Read the model definition and answer for the solid it produces. Units are mm, in the model's axes. A direction names the side the tool comes from. Give positions to 0.01 mm unless a question says otherwise; leave off trailing zeros. Order: outer loops, then holes, each group sorted by start corner. A loop starts at its lowest first (then second) coordinate and runs counter-clockwise, first axis right, second up. Notation, with made-up numbers: M 66,-30.5 L 110,-30.5 A12 ccw 110,-12.5 Z; hole C 62.25,-39 d1. An arc over 180 degrees is marked long. One line per item, written item: value.
from build123d import *

# Parameters (mm, degrees)
SKETCH2_W                                    = 325
SKETCH2_H                                    = 220
SKETCH2_R                                    = 5
BOSS_EXTRUDE3_DEPTH                          = 15
SKETCH11_W                                   = 70
SKETCH11_H                                   = 90
SKETCH11_W_2                                 = 50
SKETCH11_H_2                                 = 75
CUT_EXTRUDE6_DEPTH                           = 5
FILLET1_R                                    = 5
CSK_FOR_M4_COUNTERSUNK_FLAT_HEAD_SCR_2_COUNT = 2
CSK_FOR_M4_COUNTERSUNK_FLAT_HEAD_SCR_2_PITCH = 100
CSK_FOR_M4_COUNTERSUNK_FLAT_HEAD_SCR_3_COUNT = 2
CSK_FOR_M4_COUNTERSUNK_FLAT_HEAD_SCR_3_PITCH = 202.484567313
CSK_FOR_M4_COUNTERSUNK_FLAT_HEAD_SCR_4_COUNT = 2
CSK_FOR_M4_COUNTERSUNK_FLAT_HEAD_SCR_4_PITCH = 236.008474424
CSK_FOR_M4_COUNTERSUNK_FLAT_HEAD_SCR_5_COUNT = 2
CSK_FOR_M4_COUNTERSUNK_FLAT_HEAD_SCR_5_PITCH = 232.594066992
CSK_FOR_M4_COUNTERSUNK_FLAT_HEAD_SCR_6_COUNT = 2
CSK_FOR_M4_COUNTERSUNK_FLAT_HEAD_SCR_6_PITCH = 210
M5_TAPPED_HOLE2_D                            = 4.2
M5_TAPPED_HOLE2_DEPTH                        = 5
M5_TAPPED_HOLE2_TIP                          = 1.2618073
M6_TAPPED_HOLE3_D                            = 5
M6_TAPPED_HOLE3_DEPTH                        = 5
M6_TAPPED_HOLE3_TIP                          = 1.502151548


with BuildPart() as part:
    # Sketch2 → Boss-Extrude3 (new body)
    with BuildSketch(Plane(origin=(0, 0, 0), x_dir=(1, 0, 0), z_dir=(0, 1, 0))):
        with Locations((7.596919738, 0)):
            Rectangle(SKETCH2_W, SKETCH2_H)
        with Locations(Location((155.096919738, -95, 0), (0, 0, 270))):
            Circle(SKETCH2_R, mode=Mode.SUBTRACT)
        with Locations(Location((155.096919738, 95, 0), (0, 0, 270))):
            Circle(SKETCH2_R, mode=Mode.SUBTRACT)
        with Locations(Location((-104.903080262, -95, 0), (0, 0, 270))):
            Circle(SKETCH2_R, mode=Mode.SUBTRACT)
        with Locations(Location((-104.903080262, 95, 0), (0, 0, 90))):
            Circle(SKETCH2_R, mode=Mode.SUBTRACT)
    extrude(amount=-BOSS_EXTRUDE3_DEPTH)

    # Sketch11 → Cut-Extrude6 (cut)
    with BuildSketch(Plane.XZ.offset(15)):
        with Locations((40.096919738, -50)):
            Rectangle(SKETCH11_W, SKETCH11_H)
        with Locations((-39.903080262, -50)):
            Rectangle(SKETCH11_W, SKETCH11_H)
        with Locations((-109.903080262, -42.5)):
            Rectangle(SKETCH11_W_2, SKETCH11_H_2)
        with Locations((-109.903080262, 42.5)):
            Rectangle(SKETCH11_W_2, SKETCH11_H_2)
        with Locations((-39.903080262, 50)):
            Rectangle(SKETCH11_W, SKETCH11_H)
        with Locations((40.096919738, 50)):
            Rectangle(SKETCH11_W, SKETCH11_H)
        Polygon((85.096919738, 95), (135.096919738, 95), (140.096919738, 95), (140.096919738, 80), (155.096919738, 80), (155.096919738, 5), (85.096919738, 5), align=None)
        Polygon((85.096919738, -95), (135.096919738, -95), (140.096919738, -95), (140.096919738, -80), (155.096919738, -80), (155.096919738, -5), (85.096919738, -5), align=None)
    extrude(amount=-CUT_EXTRUDE6_DEPTH, mode=Mode.SUBTRACT)

    # Fillet1
    fillet1_edges = [part.edges().sort_by_distance(p)[0] for p in [
        (85.096919738, -12.5, -95),
        (85.096919738, -12.5, -5),
        (155.096919738, -12.5, -5),
        (155.096919738, -12.5, -80),
        (140.096919738, -12.5, -80),
        (140.096919738, -12.5, -95),
        (140.096919738, -12.5, 95),
        (140.096919738, -12.5, 80),
        (155.096919738, -12.5, 80),
        (155.096919738, -12.5, 5),
        (85.096919738, -12.5, 5),
        (75.096919738, -12.5, 5),
        (5.096919738, -12.5, 5),
        (5.096919738, -12.5, 95),
        (75.096919738, -12.5, 95),
        (-4.903080262, -12.5, 5),
        (-74.903080262, -12.5, 5),
        (-74.903080262, -12.5, 95),
        (-4.903080262, -12.5, 95),
        (-84.903080262, -12.5, 5),
        (-134.903080262, -12.5, 5),
        (-134.903080262, -12.5, 80),
        (-84.903080262, -12.5, 80),
        (-84.903080262, -12.5, -80),
        (-134.903080262, -12.5, -80),
        (-134.903080262, -12.5, -5),
        (-84.903080262, -12.5, -5),
        (-4.903080262, -12.5, -95),
        (-74.903080262, -12.5, -95),
        (-74.903080262, -12.5, -5),
        (-4.903080262, -12.5, -5),
        (75.096919738, -12.5, -95),
        (5.096919738, -12.5, -95),
        (5.096919738, -12.5, -5),
        (75.096919738, -12.5, -5),
    ]]
    fillet(fillet1_edges, radius=FILLET1_R)

    # Sketch28 → CSK for M4 Countersunk Flat Head Screw2 (revolve, cut)
    with BuildSketch(Plane(origin=(-24.903080262, -15, -105), x_dir=(0, 0, -1), z_dir=(1, 0, 0))):
        Polygon((0, 0), (0, 15), (2, 15), (2, 2.2), (3.7, 0.5), (3.7, 0), align=None)
    csk_for_m4_countersunk_flat_head_screw2 = revolve(axis=Axis((-24.903080262, -21.35, -105), (0, 1, 0)), mode=Mode.SUBTRACT)

    # CSK for M4 Countersunk Flat Head Scr 2: CSK for M4 Countersunk Flat Head Screw2 ×2
    with Locations(*[(i * CSK_FOR_M4_COUNTERSUNK_FLAT_HEAD_SCR_2_PITCH, 0, 0) for i in range(1, CSK_FOR_M4_COUNTERSUNK_FLAT_HEAD_SCR_2_COUNT)]):
        add(csk_for_m4_countersunk_flat_head_screw2, mode=Mode.SUBTRACT)

    # CSK for M4 Countersunk Flat Head Scr 3: CSK for M4 Countersunk Flat Head Screw2 ×2
    with Locations(*[Vector(0.9383431168171102, 0, 0.34570535882735626) * (i * CSK_FOR_M4_COUNTERSUNK_FLAT_HEAD_SCR_3_PITCH) for i in range(1, CSK_FOR_M4_COUNTERSUNK_FLAT_HEAD_SCR_3_COUNT)]):
        add(csk_for_m4_countersunk_flat_head_screw2, mode=Mode.SUBTRACT)

    # CSK for M4 Countersunk Flat Head Scr 4: CSK for M4 Countersunk Flat Head Screw2 ×2
    with Locations(*[Vector(0.8050558373533682, 0, 0.59319903804985) * (i * CSK_FOR_M4_COUNTERSUNK_FLAT_HEAD_SCR_4_PITCH) for i in range(1, CSK_FOR_M4_COUNTERSUNK_FLAT_HEAD_SCR_4_COUNT)]):
        add(csk_for_m4_countersunk_flat_head_screw2, mode=Mode.SUBTRACT)

    # CSK for M4 Countersunk Flat Head Scr 5: CSK for M4 Countersunk Flat Head Screw2 ×2
    with Locations(*[Vector(0.42993358039234764, 0, 0.9028605188239304) * (i * CSK_FOR_M4_COUNTERSUNK_FLAT_HEAD_SCR_5_PITCH) for i in range(1, CSK_FOR_M4_COUNTERSUNK_FLAT_HEAD_SCR_5_COUNT)]):
        add(csk_for_m4_countersunk_flat_head_screw2, mode=Mode.SUBTRACT)

    # CSK for M4 Countersunk Flat Head Scr 6: CSK for M4 Countersunk Flat Head Screw2 ×2
    with Locations(*[(0, 0, i * CSK_FOR_M4_COUNTERSUNK_FLAT_HEAD_SCR_6_PITCH) for i in range(1, CSK_FOR_M4_COUNTERSUNK_FLAT_HEAD_SCR_6_COUNT)]):
        add(csk_for_m4_countersunk_flat_head_screw2, mode=Mode.SUBTRACT)

    # M5 Tapped Hole2
    with Locations(Plane(origin=(0, 0, 0), x_dir=(1, 0, 0), z_dir=(0, 1, 0))):
        with Locations((115.096919738, 55), (115.096919738, -55), (-44.903080262, -55), (-44.903080262, 55)):
            Hole(M5_TAPPED_HOLE2_D / 2, depth=M5_TAPPED_HOLE2_DEPTH)
            with Locations((0, 0, -(M5_TAPPED_HOLE2_DEPTH + M5_TAPPED_HOLE2_TIP / 2))):  # 118° drill point
                Cone(0, M5_TAPPED_HOLE2_D / 2, M5_TAPPED_HOLE2_TIP, mode=Mode.SUBTRACT)

    # M6 Tapped Hole3
    with Locations(Plane.ZY.offset(154.903080262)):
        with Locations((-102.5, -7.5), (0, -7.5), (102.5, -7.5)):
            Hole(M6_TAPPED_HOLE3_D / 2, depth=M6_TAPPED_HOLE3_DEPTH)
            with Locations((0, 0, -(M6_TAPPED_HOLE3_DEPTH + M6_TAPPED_HOLE3_TIP / 2))):  # 118° drill point
                Cone(0, M6_TAPPED_HOLE3_D / 2, M6_TAPPED_HOLE3_TIP, mode=Mode.SUBTRACT)


solid = part.part
1) Determine the mould class of faces 1 (the face through (-40, -10, 51)), 2 (the face through (-110, -10, 43)), 3 (the face through (5, -7, -110)), 4 (the face through (170.097, -7, 2)) for opening direction Z: +Z half, -Z half, draft (parallel to the pull), parting line (faces both ways), or undercut.
Reported:
face 1: undercut
face 2: undercut
face 3: -Z half
face 4: draft
2) Which of the six approach directions +Z, -Z, +X, -X, +Y, -Y give full straight-line access (tool end or side, diameter ignored) to faces 5 (the face through (168.71, -14.75, 35.8)), 6 (the face through (153.18, -7.4, 99.62))?
Reported:
face 5: -Y
face 6: +Y, -Y
3) Find section C-C, the plane x = 126. Write down the section's boundary in (y, z).
Reported:
outline: M -15,-110 L 0,-110 L 0,110 L -15,110 L -15,95 L -10,95 L -10,5 L -15,5 L -15,-5 L -10,-5 L -10,-95 L -15,-95 Z
4) Consider probe 1 along X at (y, z) = (-5.75, 95); probe 2 along X at (y, z) = (-12.25, 71.5); probe 3 along X at (y, z) = (-1.15, 55). Determine where each line is inside the solid, lowest interval first.
Reported:
probe 1: x = -154.9 to -109.9, -99.9 to 150.1, 160.1 to 170.1
probe 2: x = -154.9 to -134.9, -84.9 to -74.9, -4.9 to 5.1, 75.1 to 85.1, 155.1 to 170.1
probe 3: x = -154.9 to -47, -42.8 to 113, 117.2 to 170.1
5) Find section B-B, the plane z = -62. Write down the section's boundary in (x, y), plus the area to 4 significant figures.
Reported:
outline: M -154.9,-15 L -134.9,-15 L -134.9,-10 L -84.9,-10 L -84.9,-15 L -74.9,-15 L -74.9,-10 L -4.9,-10 L -4.9,-15 L 5.1,-15 L 5.1,-10 L 75.1,-10 L 75.1,-15 L 85.1,-15 L 85.1,-10 L 155.1,-10 L 155.1,-15 L 170.1,-15 L 170.1,0 L -154.9,0 Z
area: 3,575 mm^2
6) Each of these flat-tipped pins is pushed along its axis until it touches: pin 1 Ø6.5 at (x, z) = (75.1, -105) entering from -Y; pin 2 Ø4 at (x, z) = (-44.9, -55) entering from -Y; pin 3 Ø2.5 at (x, z) = (75.1, 105) entering from -Y. Where does it stop, or does it pass through?
Reported:
pin 1: stops at y = -14.05
pin 2: stops at y = -10
pin 3: passes through
7) Find section A-A, the plane x = -94. Write down the section's boundary in (y, z).
Reported:
outline: M -15,-110 L 0,-110 L 0,110 L -15,110 L -15,80 L -10,80 L -10,5 L -15,5 L -15,-5 L -10,-5 L -10,-80 L -15,-80 Z
